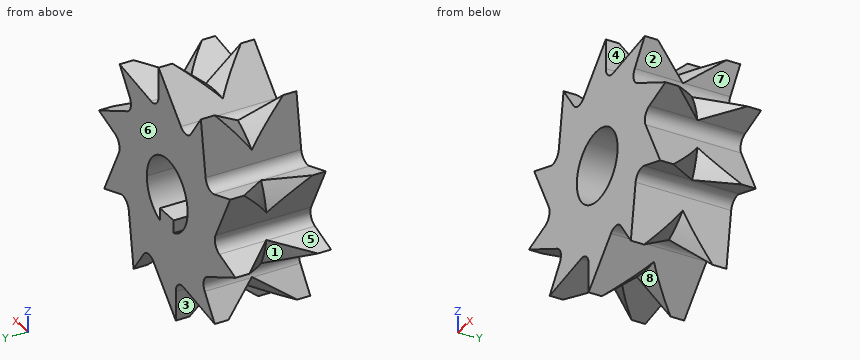
```python
from build123d import *

# Parameters (mm, degrees)
F1_DEPTH = 42.926
F2_R     = 5.08
F5_DEPTH = 24.384
F6_R     = 5.08


with BuildPart() as f1:
    # F0 (on Front) → F1 (new body)
    with BuildSketch(Plane.XZ):
        Polygon((6.703672, 53.90551), (-14.948268, 31.979494), (-26.26148, 47.550793), (-30.890478, 17.085582), (-49.195638, 23.033289), (-35.033575, -4.334441), (-53.338735, -10.282148), (-25.795037, -24.098855), (-37.108248, -39.670155), (-6.703672, -34.658326), (-6.703672, -53.90551), (14.948268, -31.979494), (26.26148, -47.550793), (30.890478, -17.085582), (49.195638, -23.033289), (35.033575, 4.334441), (53.338735, 10.282148), (25.795037, 24.098855), (37.108248, 39.670155), (6.703672, 34.658326), align=None)
        with BuildLine():
            ThreePointArc((-5.035342, -15.090275), (-9.299672, 12.906865), (15.908207, 0))
            ThreePointArc((15.908207, 0), (13.090102, -9.039928), (5.634228, -14.877047))
            ThreePointArc((5.634228, -14.877047), (0.317856, -15.905032), (-5.035342, -15.090275))
        make_face(mode=Mode.SUBTRACT)
    extrude(amount=F1_DEPTH)

    # F2
    f2_edges = [f1.edges().sort_by_distance(p)[0] for p in [
        (25.795037, -21.463, 24.098855),
        (6.703672, -21.463, 34.658326),
        (35.033575, -21.463, 4.334441),
        (30.890478, -21.463, -17.085582),
        (14.948268, -21.463, -31.979494),
        (-6.703672, -21.463, -34.658326),
        (-25.795037, -21.463, -24.098855),
        (-35.033575, -21.463, -4.334441),
        (-30.890478, -21.463, 17.085582),
        (-14.948268, -21.463, 31.979494),
    ]]
    fillet(f2_edges, radius=F2_R)

    # F3 (on Right) → F4 (revolve, cut)
    with BuildSketch(Plane.YZ):
        Polygon((-6.094482, 54.397043), (-37.077803, 54.397043), (-21.222165, 40.98073), align=None)
    revolve(axis=Axis((0, -28.662119, 0), (0, 1, 0)), mode=Mode.SUBTRACT)

    # F0 (on Front) → F5 (join)
    with BuildSketch(Plane.XZ):
        with BuildLine():
            Line((-5.035342, -9.313321), (-5.035342, -15.090275))
            ThreePointArc((-5.035342, -15.090275), (0.317856, -15.905032), (5.634228, -14.877047))
            Line((5.634228, -14.877047), (5.634228, -9.313321))
            Line((5.634228, -9.313321), (-5.035342, -9.313321))
        make_face()
    extrude(amount=F5_DEPTH)

    # F6
    f6_edges = [f1.edges().sort_by_distance(p)[0] for p in [
        (5.634228, -24.384, -12.095184),
        (-5.035342, -24.384, -12.201798),
    ]]
    fillet(f6_edges, radius=F6_R)


solid = f1.part
```
Geometry check sheet. Reference: the model listing, model coordinates, mm. Face numbers are marked on the shaded views. A direction names the side the tool comes from. Coordinates: 2 decimals unless noted, no trailing zeros. Write each loop counter-clockwise with the first axis right and the second up, starting at its lowest first coordinate (ties: lowest second). Pieces come first, ordered by that corner, then holes. Notation, with made-up numbers: M 51.5,15 L 94.5,15 A15 cw 94.5,43 Z; hole C 4.25,8.25 d3. An arc over 180 degrees is marked long. Use one line per item in the form item = value. Start each with the question number.
1) Section check C-C on x = -44. State how many separate pieces and enclosed holes the cut face has, and give its area (3 significant figures).
2) Release check for a two-part mould opening along Z. For the marked faces 6, 7 and 8 record: pulls with the +Z half, pulls with the -Z half, needs draft (parallel to the pull), parting line crosses it, or undercut.
3) Section check B-B on z = -3. Enter the section's corners in (x, y), and give its area (3 significant figures).
4) Set-up check for the marked faces 1, 2, 3, 4 and 5: record each of +Z, -Z, +X, -X, +Y, -Y from which the full face is reachable in a straight line by a thin tool's end or side.
5) Go/stop test with flat-tipped pins: pin 1 Ø5.5 at (x, y) = (1, -16) entering from +Z; pin 2 Ø6.5 at (y, z) = (-11, -13.5) entering from -X; pin 3 Ø2 at (x, y) = (33, -29) entering from -Z. Record where each tip stops, or that it passes through.
6) Thickness scan on probe 1 along X at (y, z) = (-27, 0); probe 2 along Z at (x, y) = (0, -17); probe 3 along Z at (x, y) = (-13.5, -15.5). Record the ranges inside material, lowest first. Write a range as from..to.
Responses:
q1.separate_pieces = 4
q1.enclosed_holes = 0
q1.area = 489 mm2
q2.face_6 = needs draft
q2.face_7 = undercut
q2.face_8 = pulls with the -Z half
q3.outline = M -37.49,-42.93 L -15.62,-42.93 L -15.62,0 L -37.49,0 Z; M 15.62,-42.93 L 38.83,-42.93 L 38.83,0 L 15.62,0 Z
q3.area = 1,930 mm2
q4.face_1 = -Z, -X
q4.face_2 = +X, +Y, -Y
q4.face_3 = -Z, -X, +Y, -Y
q4.face_4 = +Z, +X, +Y, -Y
q4.face_5 = -X, +Y, -Y
q5.pin_1 = 48.04
q5.pin_2 = -51.01
q5.pin_3 = -19.68
q6.probe_1 = -37.4..-15.91, 15.91..37.4
q6.probe_2 = -44.73..-9.31, 15.91..44.73
q6.probe_3 = -35.78..-8.42, 8.42..34.8
